Model file for the job. Use its own axes, mm. A direction names the side the tool comes from. Round coordinates to 2 decimals unless told otherwise and drop trailing zeros. Loops run counter-clockwise (first coordinate to the right, second up) from the corner with the lowest first, then second, coordinate; pieces in that order, holes last. Notation, with made-up numbers: M -36,15 L -31,15 A16 ccw -31,40 Z; hole C -28.75,44.5 d9. An arc over 180 degrees is marked long. Use a Markdown table: item, result. Add a question column.
Q1. Pin check, flat tips, straight feed: pin 1 (2 mm diameter, centred on x = -62, y = 70.5, fed in from -Z); pin 2 (12 mm diameter, centred on y = 60.5, z = 38.5, fed in from +X); pin 3 (2 mm diameter, centred on x = 52, y = 54.5, fed in from +Z). Stop position of each tip, or through.
Q2. Cut at D-D (x = -49). Give the cut face in (y, z), plus the area to 3 significant figures.
Q3. Probe line 1 (Y direction, x = 83.25, z = 0); line 2 (Y direction, x = 0, z = -85); line 3 (X direction, y = 58.5, z = 51.5). List the from-to ranges inside material, lowest first. Write a range as from..to.
Q4. Cut at B-B (x = 0). Give the cut face in (y, z).
Q5. Cut at C-C (z = 70.5). Give the cut face in (x, y).
Q6. Mould opens along Z. For faces 1 (the face through (76.255, 39.44, 31.617)), 2 (the face through (82.12, 39.44, 34.05)), 3 (the face through (26, 80, 79)) say: +Z half, -Z half, draft (parallel to the pull), parting line (faces both ways), or undercut.
Q7. Tool access for faces 4 (the face through (84.1, 43.49, -12.1)), 5 (the face through (-84.096, 43.308, -12.096)), 6 (the face through (26, 0, 79)): list every direction of +Z, -Z, +X, -X, +Y, -Y with a clear straight run to the whole face (end or side of a thin tool).
Q8. Cut at A-A (z = 0). Give the cut face in (x, y).
from build123d import *

# Parameters (mm, degrees)
SKETCH1_R           = 88.9
BOSS_EXTRUDE1_DEPTH = 80
SKETCH2_R           = 82.55
CUT_EXTRUDE4_DEPTH  = 90
SKETCH12_R          = 22.5
CUT_EXTRUDE5_DEPTH  = 115.64
SKETCH13_R          = 22.5
CUT_EXTRUDE6_DEPTH  = 115.64
SKETCH14_R          = 22.5
CUT_EXTRUDE7_DEPTH  = 99.64
SKETCH15_R          = 22.5
CUT_EXTRUDE8_DEPTH  = 137.64


with BuildPart() as part:
    # Sketch1 → Boss-Extrude1 (new body)
    with BuildSketch(Plane(origin=(0, 0, 0), x_dir=(1, 0, 0), z_dir=(0, 1, 0))):
        Circle(SKETCH1_R)
    extrude(amount=BOSS_EXTRUDE1_DEPTH)

    # Sketch2 → Cut-Extrude4 (cut)
    with BuildSketch(Plane(origin=(0, 0, 0), x_dir=(1, 0, 0), z_dir=(0, 1, 0))):
        Circle(SKETCH2_R)
    extrude(amount=CUT_EXTRUDE4_DEPTH, mode=Mode.SUBTRACT)

    # Sketch12 → Cut-Extrude5 (cut)
    with BuildSketch(Plane(origin=(0, 0, 0), x_dir=(0, 0, -1), z_dir=(1, 0, 0))):
        with Locations((0, 24.336091646)):
            Circle(SKETCH12_R)
    extrude(amount=-CUT_EXTRUDE5_DEPTH, mode=Mode.SUBTRACT)

    # Sketch13 → Cut-Extrude6 (cut)
    with BuildSketch(Plane.XY):
        with Locations((0, 25.450721797)):
            Circle(SKETCH13_R)
    extrude(amount=-CUT_EXTRUDE6_DEPTH, mode=Mode.SUBTRACT)

    # Sketch14 → Cut-Extrude7 (cut)
    with BuildSketch(Plane(origin=(0, 0, 0), x_dir=(0, 0, -1), z_dir=(1, 0, 0))):
        with Locations((0, 24.521863338)):
            Circle(SKETCH14_R)
    extrude(amount=CUT_EXTRUDE7_DEPTH, mode=Mode.SUBTRACT)

    # Sketch15 → Cut-Extrude8 (cut)
    with BuildSketch(Plane.XY):
        with Locations((0, 25.450721797)):
            Circle(SKETCH15_R)
    extrude(amount=CUT_EXTRUDE8_DEPTH, mode=Mode.SUBTRACT)


solid = part.part
Checked values:
| question | item | result |
|---|---|---|
| 1 | pin 1 | stops at z = -64.67 |
| 1 | pin 2 | stops at x = 82.75 |
| 1 | pin 3 | stops at z = 72.82 |
| 2 | outline | M 0,-74.18 L 80,-74.18 L 80,-66.43 L 0,-66.43 Z; M 0,66.43 L 80,66.43 L 80,74.18 L 0,74.18 Z |
| 2 | area | 1,240 mm^2 |
| 3 | line 1 | y = 0..2.02, 47.02..80 |
| 3 | line 2 | y = 0..2.95, 47.95..80 |
| 3 | line 3 | x = -72.46..-64.52, 64.52..72.46 |
| 4 | outline | M 0,-88.9 L 2.95,-88.9 L 2.95,-82.55 L 0,-82.55 Z; M 0,82.55 L 2.95,82.55 L 2.95,88.9 L 0,88.9 Z; M 47.95,-88.9 L 80,-88.9 L 80,-82.55 L 47.95,-82.55 Z; M 47.95,82.55 L 80,82.55 L 80,88.9 L 47.95,88.9 Z |
| 5 | outline | M -54.16,0 L -42.94,0 L -42.94,80 L -54.16,80 Z; M 42.94,0 L 54.16,0 L 54.16,80 L 42.94,80 Z |
| 6 | face 1 | undercut |
| 6 | face 2 | parting line |
| 6 | face 3 | draft |
| 7 | face 4 | +X |
| 7 | face 5 | -X |
| 7 | face 6 | +Z, -Z, +X, -X, -Y |
| 8 | outline | M -88.9,0 L -82.55,0 L -82.55,1.84 L -88.9,1.84 Z; M -88.9,46.84 L -82.55,46.84 L -82.55,80 L -88.9,80 Z; M 82.55,0 L 88.9,0 L 88.9,2.02 L 82.55,2.02 Z; M 82.55,47.02 L 88.9,47.02 L 88.9,80 L 82.55,80 Z |
